Study the drawing (mm; zero at the part's minimum x, y, z) and answer. A direction names the side the tool comes from. Coordinates: 2 decimals unless noted, no trailing zeros. Order: outer loops, then holes, each group sorted by start corner. A loop starts at its lowest first (then second) coordinate and runs counter-clockwise, first axis right, second up. Notation, with made-up numbers: (-38, 62) - (-28, 62) arc R18 ccw to (-28, 93) - close; hole circle Ø4 at (-17, 14). An arc over 180 degrees is marked (long way). Write item = value, one per line.
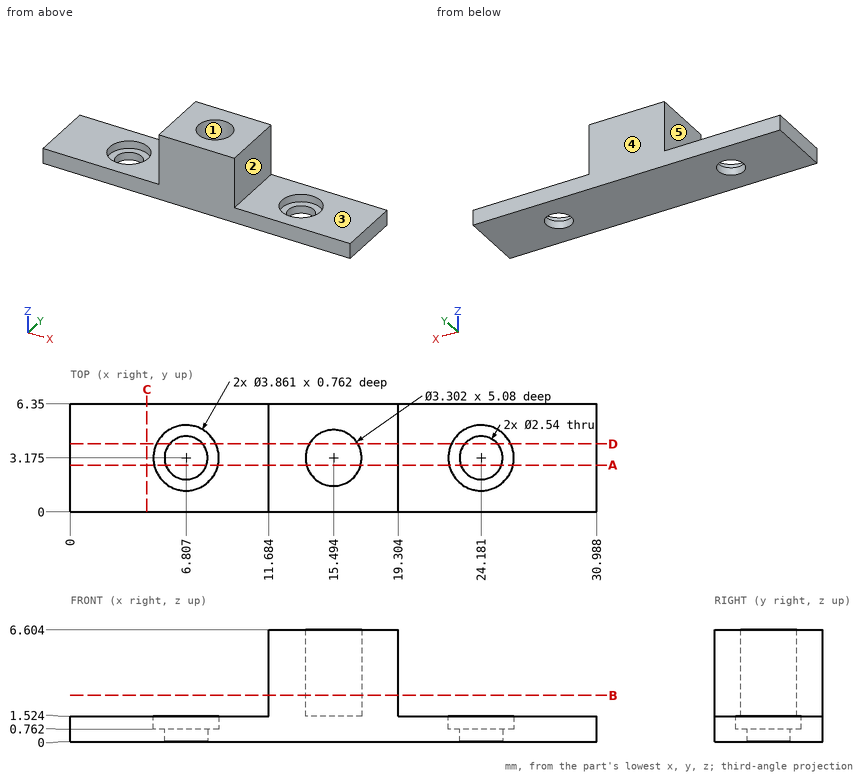
1) Determine the mould class of the marked faces 1, 2 and 3 for opening direction X: pulls with the +X half, pulls with the -X half, needs draft (parallel to the pull), parting line crosses it, or undercut.
Returned:
face_1 = undercut
face_2 = pulls with the +X half
face_3 = needs draft
2) For the marked faces 4 and 5, determine the directions among +Z, -Z, +X, -X, +Y, -Y from which every point of the face is accessible in a straight line to the end or side of a thin tool.
Returned:
face_4 = +Z, -Z, +X, -X, +Y
face_5 = +Z, -X, +Y, -Y
3) The part is cut by section A-A (y = 2.75). Determine the outline of the cut face in (x, z).
Returned:
outline = (0, 0) - (5.61, 0) - (5.61, 0.76) - (4.92, 0.76) - (4.92, 1.52) - (0, 1.52) - close; (8, 0) - (22.98, 0) - (22.98, 0.76) - (22.3, 0.76) - (22.3, 1.52) - (19.3, 1.52) - (19.3, 6.6) - (17.09, 6.6) - (17.09, 1.52) - (13.9, 1.52) - (13.9, 6.6) - (11.68, 6.6) - (11.68, 1.52) - (8.69, 1.52) - (8.69, 0.76) - (8, 0.76) - close; (25.38, 0) - (30.99, 0) - (30.99, 1.52) - (26.06, 1.52) - (26.06, 0.76) - (25.38, 0.76) - close
4) The part is cut by section B-B (z = 2.75). Determine the outline of the cut face in (x, y) (3 decimals), and give its area (3 significant figures).
Returned:
outline = (11.684, 0) - (19.304, 0) - (19.304, 6.35) - (11.684, 6.35) - close; hole circle Ø3.302 at (15.494, 3.175)
area = 39.8 mm^2
5) Straight lines are drawn through the part: line 1 along X through (y, z) = (3.25, 1); line 2 along Z through (x, y) = (16, 4.25); line 3 along Z through (x, y) = (22.5, 2.75). For each, find the intervals that lie inside material, in ascending order. Write a range as from..to.
Returned:
line_1 = 0..4.88, 8.74..22.25, 26.11..30.99
line_2 = 0..1.52
line_3 = 0..0.76
6) The part is cut by section D-D (y = 4). Determine the outline of the cut face in (x, z) (1 decimal).
Returned:
outline = (0, 0) - (5.8, 0) - (5.8, 0.8) - (5.1, 0.8) - (5.1, 1.5) - (0, 1.5) - close; (7.8, 0) - (23.2, 0) - (23.2, 0.8) - (22.4, 0.8) - (22.4, 1.5) - (19.3, 1.5) - (19.3, 6.6) - (16.9, 6.6) - (16.9, 1.5) - (14.1, 1.5) - (14.1, 6.6) - (11.7, 6.6) - (11.7, 1.5) - (8.6, 1.5) - (8.6, 0.8) - (7.8, 0.8) - close; (25.1, 0) - (31, 0) - (31, 1.5) - (25.9, 1.5) - (25.9, 0.8) - (25.1, 0.8) - close
7) The part is cut by section C-C (x = 4.5). Determine the outline of the cut face in (y, z).
Returned:
outline = (0, 0) - (6.35, 0) - (6.35, 1.52) - (0, 1.52) - close
8) Flat-ended cylindrical pins translate along their axes: pin 1 Ø1.7 at (x, y) = (15.5, 3.5) entering from +Z; pin 2 Ø3 at (x, y) = (7, 3) entering from +Z; pin 3 Ø1.5 at (y, z) = (3.5, 3) entering from +X. Find the tip coordinate at first contact, or state that the pin passes through.
Returned:
pin_1 = 1.52
pin_2 = 0.76
pin_3 = 19.3
